from build123d import *

# Parameters (mm, degrees)
ESQUISSE1_R        = 2.975
ESQUISSE1_R_2      = 1.5
BOSS_EXTRU_1_DEPTH = 5
ESQUISSE2_R        = 0.26
BOSS_EXTRU_2_DEPTH = 5


with BuildPart() as part:
    # Esquisse1 → Boss.-Extru.1 (new body)
    with BuildSketch(Plane.XY):
        with BuildLine():
            Line((0.125901786, 5.973673387), (70.094821429, 4.499000878))
            ThreePointArc((70.094821429, 4.499000878), (74.5, 0), (70.094821429, -4.499000878))
            Line((70.094821429, -4.499000878), (0.125901786, -5.973673387))
            ThreePointArc((0.125901786, -5.973673387), (-5.975, 0), (0.125901786, 5.973673387))
        make_face()
        Circle(ESQUISSE1_R, mode=Mode.SUBTRACT)
        with Locations((70, 0)):
            Circle(ESQUISSE1_R_2, mode=Mode.SUBTRACT)
    extrude(amount=BOSS_EXTRU_1_DEPTH)

    # Esquisse2 → Boss.-Extru.2 (add)
    with BuildSketch(Plane.XY.offset(5)):
        with Locations((2.951541236, 0.37286637)):
            Circle(ESQUISSE2_R)
        with Locations((2.951541236, -0.37286637)):
            Circle(ESQUISSE2_R)
        with Locations((2.766085046, -1.095170544)):
            Circle(ESQUISSE2_R)
        with Locations((2.406825558, -1.748661126)):
            Circle(ESQUISSE2_R)
        with Locations((1.89633637, -2.292276897)):
            Circle(ESQUISSE2_R)
        with Locations((1.266693392, -2.691860481)):
            Circle(ESQUISSE2_R)
        with Locations((0.557459411, -2.922304571)):
            Circle(ESQUISSE2_R)
        with Locations((-0.186801796, -2.969129517)):
            Circle(ESQUISSE2_R)
        with Locations((-0.919325558, -2.829393136)):
            Circle(ESQUISSE2_R)
        with Locations((-1.594084715, -2.511875578)):
            Circle(ESQUISSE2_R)
        with Locations((-2.168681667, -2.03652764)):
            Circle(ESQUISSE2_R)
        with Locations((-2.607012373, -1.43321718)):
            Circle(ESQUISSE2_R)
        with Locations((-2.881534904, -0.739852414)):
            Circle(ESQUISSE2_R)
        with Locations((-2.975, 0)):
            Circle(ESQUISSE2_R)
        with Locations((-2.881534904, 0.739852414)):
            Circle(ESQUISSE2_R)
        with Locations((-2.607012373, 1.43321718)):
            Circle(ESQUISSE2_R)
        with Locations((-2.168681667, 2.03652764)):
            Circle(ESQUISSE2_R)
        with Locations((-1.594084715, 2.511875578)):
            Circle(ESQUISSE2_R)
        with Locations((-0.919325558, 2.829393136)):
            Circle(ESQUISSE2_R)
        with Locations((-0.186801796, 2.969129517)):
            Circle(ESQUISSE2_R)
        with Locations((0.557459411, 2.922304571)):
            Circle(ESQUISSE2_R)
        with Locations((1.266693392, 2.691860481)):
            Circle(ESQUISSE2_R)
        with Locations((1.89633637, 2.292276897)):
            Circle(ESQUISSE2_R)
        with Locations((2.406825558, 1.748661126)):
            Circle(ESQUISSE2_R)
        with Locations((2.766085046, 1.095170544)):
            Circle(ESQUISSE2_R)
    extrude(amount=-BOSS_EXTRU_2_DEPTH)


solid = part.part
Geometry check sheet. Reference: the model listing, model coordinates, mm. Give positions to 0.01 mm unless a question says otherwise; leave off trailing zeros. Loops run counter-clockwise (first coordinate to the right, second up) from the corner with the lowest first, then second, coordinate; pieces in that order, holes last. Notation, with made-up numbers: (-8, 4.5) -> (29, 4.5) arc R29 cw to (29, 39.5) -> close; hole circle Ø3 at (27, -11.75). An arc over 180 degrees is marked (long way). Answer in a Markdown table with one row per item. Add a question column.
1) Gauge pin test, flat ends, axial feed: P1, Ø2.5, axis at x = 70, y = 0, coming from the -Z side; P2, Ø3, axis at y = -3, z = 2, coming from the +X side; P3, Ø1, axis at y = 3.5, z = 1, coming from the -X side. Record the tip position at first contact, or that the pin passes through.
2) Cross-section at C-C on x = 5.5. Record the boundary of the cut face in (y, z).
3) Draft check along X on faces 1 (the face through (35, 0, 0)), 2 (the face through (74.5, 0.1, 2.5)), 3 (the face through (71.43, 0.45, 2.46)). Enter one of: pulls with the +X half, pulls with the -X half, needs draft (parallel to the pull), parting line crosses it, or undercut.
4) Cross-section at A-A on z = 2. State how many separate pieces and enclosed holes the cut face has, and give its area (3 significant figures).
5) Material ranges on probe 1 along Y at (x, z) = (70, 2.9); probe 2 along X at (y, z) = (1, 1.2); probe 3 along X at (y, z) = (0.75, 2.7), recorded low to high. Write a range as from..to.
6) Cross-section at B-B on x = 52.5. Record the boundary of the cut face in (y, z).
Outcome:
| question | item | result |
|---|---|---|
| 1 | P1 | passes through |
| 1 | P2 | stops at x = 74.24 |
| 1 | P3 | stops at x = -5.17 |
| 2 | outline | (-5.86, 0) -> (5.86, 0) -> (5.86, 5) -> (-5.86, 5) -> close |
| 3 | face 1 | needs draft |
| 3 | face 2 | pulls with the +X half |
| 3 | face 3 | undercut |
| 4 | separate pieces | 1 |
| 4 | enclosed holes | 2 |
| 4 | area | 789 mm^2 |
| 5 | probe 1 | y = -4.5..-1.5, 1.5..4.5 |
| 5 | probe 2 | x = -5.89..-2.8, 2.52..68.88, 71.12..74.39 |
| 5 | probe 3 | x = -5.93..-2.62, 2.88..68.7, 71.3..74.44 |
| 6 | outline | (-4.87, 0) -> (4.87, 0) -> (4.87, 5) -> (-4.87, 5) -> close |
